Autodesk Inventor part; units mm, degrees
ref_plane "YZ Plane" through (0, 0, 0) normal (1, 0, 0) x (0, 1, 0)
ref_plane "XZ Plane" through (0, 0, 0) normal (0, 1, 0) x (-1, 0, 0)
ref_plane "XY Plane" through (0, 0, 0) normal (0, 0, 1) x (1, 0, 0)
sketch "Эскиз1" plane through (0, 0, 0) normal (0, 1, 0) x (-1, 0, 0)
  line L0 (-53.5804, -13.9309) -> (-0.75, -0.195)
  line L1 (-52.3223, -18.77) -> (-0.75, -5.3612)
  line L2 (-55.3709, -15.7214) -> (-55.3709, -16.9796)
  circle A0 centre (-52.9514, -16.3505) radius 1.65
  line L3 (-0.75, -5.3612) -> (-0.75, -0.195)
  arc A1 (-55.3709, -16.9796) -> (-52.3223, -18.77) centre (-52.9514, -16.3505) ccw
  arc A2 (-53.5804, -13.9309) -> (-55.3709, -15.7214) centre (-52.9514, -16.3505) ccw
  point P0 (0, 0)
extrude "Выдавливание1" add sketch "Эскиз1" along normal blind 24
sketch "Эскиз24" plane through (0, 24, 0) normal (0, 1, 0) x (1, 0, 0)
  circle A0 centre (52.9514, 16.3505) radius 1.65
  line L0 (52.9514, 16.3505) -> (43.2731, 13.8341)
  circle A1 centre (43.2731, 13.8341) radius 1.65
  circle A2 centre (38.434, 12.576) radius 1.65
  line L1 (48.1122, 15.0923) -> (38.434, 12.576)
  circle A3 centre (33.5949, 11.3178) radius 1.65
  line L2 (43.2731, 13.8341) -> (33.5949, 11.3178)
  circle A4 centre (28.7558, 10.0596) radius 1.65
  line L3 (38.434, 12.576) -> (28.7558, 10.0596)
  circle A5 centre (23.9167, 8.8015) radius 1.65
  line L4 (33.5949, 11.3178) -> (23.9167, 8.8015)
  circle A6 centre (19.0776, 7.5433) radius 1.65
  line L5 (28.7558, 10.0596) -> (19.0776, 7.5433)
  point P0 (0, 0)
  dimension "d126" = 3.3
  dimension "d129" = 5
extrude "Выдавливание24" cut sketch "Эскиз24" against normal blind 3 contours A6 | A5 L5 L4 | L4 L5 A5 | A4 L4 L3 | L3 L4 A4 | A3 L3 L2 | L2 L3 A3 | A2 L2 L1 | L1 L2 A2 | A1 L1 L0 | L0 L1 A1
sketch "Эскиз25" plane through (19.0776, 21, -7.5433) normal (0, 1, 0) x (1, 0, 0)
  circle A0 centre (0, 0) radius 1.65
  circle A1 centre (0, 0) radius 1.15
  circle A2 centre (4.8391, 1.2582) radius 1.65
  circle A3 centre (4.8391, 1.2582) radius 1.15
  circle A4 centre (9.6782, 2.5163) radius 1.65
  circle A5 centre (9.6782, 2.5163) radius 1.15
  circle A6 centre (14.5173, 3.7745) radius 1.65
  circle A7 centre (14.5173, 3.7745) radius 1.15
  circle A8 centre (19.3565, 5.0327) radius 1.65
  circle A9 centre (19.3565, 5.0327) radius 1.15
  circle A10 centre (24.1956, 6.2908) radius 1.65
  circle A11 centre (24.1956, 6.2908) radius 1.15
  point P0 (-19.0776, -7.5433)
  dimension "d136" = 2.3
  dimension "d137" = 2.3
  dimension "d138" = 2.3
  dimension "d139" = 2.3
  dimension "d140" = 2.3
  dimension "d141" = 2.3
extrude "Выдавливание25" cut sketch "Эскиз25" against normal blind 5 contours A1 | A3 | A5 | A7 | A9 | A11
properties part number "only_top_gate"
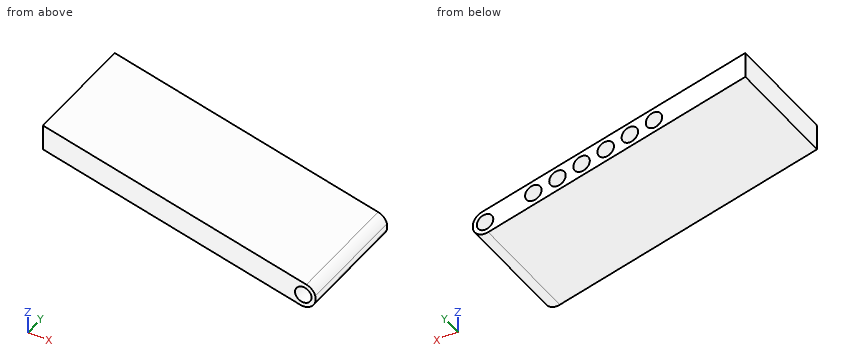
Part model, mm, in its own coordinate system. Give positions to 0.01 mm unless a question says otherwise; leave off trailing zeros. Order: outer loops, then holes, each group sorted by start corner. A loop starts at its lowest first (then second) coordinate and runs counter-clockwise, first axis right, second up. Notation, with made-up numbers: M 58,-24.5 L 77,-24.5 A23 ccw 77,1.5 Z; hole C -30,-9.75 d2. An arc over 180 degrees is marked long. Use a Markdown table: item, result. Add a question column.
(1) Drop flat-ended pins along their axis: P1, Ø3, axis at x = 29, y = 21, coming from the +Z side; P2, Ø1.6, axis at x = 23.5, z = -8.5, coming from the +Y side; P3, Ø1.8, axis at x = 43.27, z = -13.83, coming from the +Y side. Give the stop position or say it passes through.
(2) Saw through at C-C, the plane z = -4. Give the cut face in (x, y), and give its area (3 significant figures).
(3) Saw through at B-B, the plane x = 29. Give the cut face in (y, z), and give its area (3 significant figures).
(4) Saw through at D-D, the plane x = 23.5. Give the cut face in (y, z), and give its area (3 significant figures).
(5) Probe line 1 along Z through (x, y) = (34.5, 17.25); line 2 along Z through (x, y) = (37.5, 20); line 3 along Z through (x, y) = (40, 14.5). List the from-to ranges inside material, lowest first. Write a range as [from, to].
Answer key:
| question | item | result |
|---|---|---|
| 1 | P1 | z = -7.15 |
| 1 | P2 | y = 21 |
| 1 | P3 | y = 16 |
| 2 | outline | M 0.75,0 L 15.38,0 L 15.38,24 L 0.75,24 Z |
| 2 | area | 351 mm^2 |
| 3 | outline | M 0,-12.71 L 24,-12.71 L 24,-11.69 L 21,-11.69 L 21,-11.18 L 16,-11.18 L 16,-8.94 L 21,-8.94 L 21,-8.43 L 24,-8.43 L 24,-7.54 L 0,-7.54 Z |
| 3 | area | 103 mm^2 |
| 4 | outline | M 0,-11.28 L 24,-11.28 L 24,-10.4 L 21,-10.4 L 21,-9.87 L 16,-9.87 L 16,-7.73 L 21,-7.73 L 21,-7.2 L 24,-7.2 L 24,-6.11 L 0,-6.11 Z |
| 4 | area | 104 mm^2 |
| 5 | line 1 | [-14.14, -12.03], [-10.61, -8.97] |
| 5 | line 2 | [-14.92, -13.25], [-11.91, -9.75] |
| 5 | line 3 | [-15.57, -10.4] |
